Input: part model. Units: mm. Frame: model coordinates. Face numbers are marked on the shaded views. A direction names the side the tool comes from. Give positions to 0.01 mm unless a question says otherwise; leave off trailing zeros. Loops run counter-clockwise (first coordinate to the right, second up) from the corner with the lowest first, then second, coordinate; pieces in that order, holes last. Notation, with made-up numbers: (86.5, 51) - (139.5, 51) arc R23 cw to (139.5, 66) - close; hole circle Ø1 at (-29.75, 35). An arc over 180 degrees is marked (long way). One line per item, written item: value.
from build123d import *

# Parameters (mm, degrees)
SKETCH_1_W             = 80
SKETCH_1_H             = 80
EXTRUDE_1_DEPTH        = 12
HOLE_WIZARD_M161_D     = 14
HOLE_WIZARD_M161_DEPTH = 12
SKETCH_12_R            = 4.5
CUT_EXTRUDE_1_DEPTH    = 13
SKETCH_13_R            = 7.5
CUT_EXTRUDE_2_DEPTH    = 9


with BuildPart() as part:
    # Эскиз1 → Бобышка-Вытянуть1 (new body)
    with BuildSketch(Plane(origin=(0, 0, 0), x_dir=(1, 0, 0), z_dir=(0, 1, 0))):
        Rectangle(SKETCH_1_W, SKETCH_1_H)
    extrude(amount=EXTRUDE_1_DEPTH)

    # Отверстие обработанное метчиком M161
    with Locations(Plane(origin=(0, 12, 0), x_dir=(1, 0, 0), z_dir=(0, 1, 0))):
        with Locations((0, 0)):
            Hole(HOLE_WIZARD_M161_D / 2, depth=HOLE_WIZARD_M161_DEPTH)

    # Эскиз12 → Вырез-Вытянуть1 (cut, through all)
    with BuildSketch(Plane(origin=(0, 12, 0), x_dir=(1, 0, 0), z_dir=(0, 1, 0))):
        with Locations(Location((-20, 20, 0), (0, 0, 270))):  # turned: the seam where the file's is
            Circle(SKETCH_12_R)
        with Locations(Location((20, 20, 0), (0, 0, 270))):  # turned: the seam where the file's is
            Circle(SKETCH_12_R)
        with Locations(Location((20, -20, 0), (0, 0, 270))):  # turned: the seam where the file's is
            Circle(SKETCH_12_R)
        with Locations(Location((-20, -20, 0), (0, 0, 270))):  # turned: the seam where the file's is
            Circle(SKETCH_12_R)
    extrude(amount=-CUT_EXTRUDE_1_DEPTH, mode=Mode.SUBTRACT)

    # Эскиз13 → Вырез-Вытянуть2 (cut)
    with BuildSketch(Plane(origin=(0, 12, 0), x_dir=(1, 0, 0), z_dir=(0, 1, 0))):
        with Locations(Location((-20, 20, 0), (0, 0, 270))):  # turned: the seam where the file's is
            Circle(SKETCH_13_R)
        with Locations(Location((20, 20, 0), (0, 0, 270))):  # turned: the seam where the file's is
            Circle(SKETCH_13_R)
        with Locations(Location((20, -20, 0), (0, 0, 270))):  # turned: the seam where the file's is
            Circle(SKETCH_13_R)
        with Locations(Location((-20, -20, 0), (0, 0, 270))):  # turned: the seam where the file's is
            Circle(SKETCH_13_R)
    extrude(amount=-CUT_EXTRUDE_2_DEPTH, mode=Mode.SUBTRACT)


solid = part.part
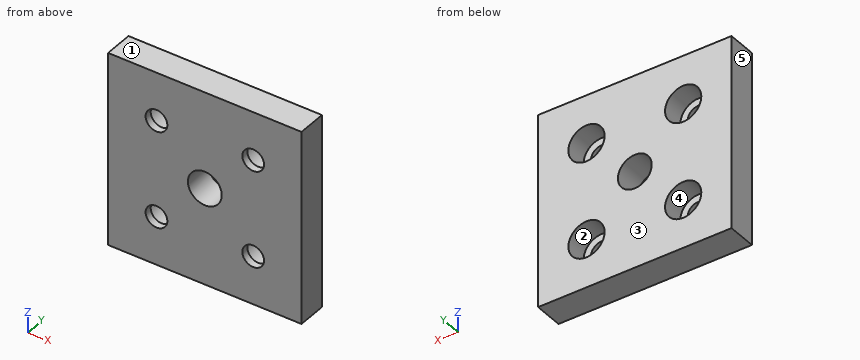
Item 1: Section A-A, the plane z = -20. Output: boundary loops of the cut face in (x, y).
Verdict:
outline: (-40, 0) - (-24.5, 0) - (-24.5, 3) - (-27.5, 3) - (-27.5, 12) - (-40, 12) - close; (-15.5, 0) - (15.5, 0) - (15.5, 3) - (12.5, 3) - (12.5, 12) - (-12.5, 12) - (-12.5, 3) - (-15.5, 3) - close; (24.5, 0) - (40, 0) - (40, 12) - (27.5, 12) - (27.5, 3) - (24.5, 3) - close
Item 2: Pin query (flat end, axial travel): P1, Ø4.5, axis at x = -23, z = 16.5, coming from the +Y side; P2, Ø1, axis at x = -3.5, z = 27.5, coming from the -Y side. Return the tip coordinate at first contact, or that it passes through.
Verdict:
P1: stops at y = 3
P2: stops at y = 0
Item 3: Section D-D, the plane z = 0. Output: boundary loops of the cut face in (x, y), and give its area (3 significant figures).
Verdict:
outline: (-40, 0) - (-7, 0) - (-7, 12) - (-40, 12) - close; (7, 0) - (40, 0) - (40, 12) - (7, 12) - close
area: 792 mm^2
Item 4: Section B-B, the plane x = 20. Output: boundary loops of the cut face in (y, z).
Verdict:
outline: (0, -40) - (12, -40) - (12, -27.5) - (3, -27.5) - (3, -24.5) - (0, -24.5) - close; (0, -15.5) - (3, -15.5) - (3, -12.5) - (12, -12.5) - (12, 12.5) - (3, 12.5) - (3, 15.5) - (0, 15.5) - close; (0, 24.5) - (3, 24.5) - (3, 27.5) - (12, 27.5) - (12, 40) - (0, 40) - close
Item 5: Section C-C, the plane y = 6. Output: boundary loops of the cut face in (x, z), and give its area (3 significant figures).
Verdict:
outline: (-40, -40) - (40, -40) - (40, 40) - (-40, 40) - close; hole circle Ø15 at (-20, -20); hole circle Ø15 at (-20, 20); hole circle Ø14 at (0, 0); hole circle Ø15 at (20, -20); hole circle Ø15 at (20, 20)
area: 5,540 mm^2
Item 6: Material intervals for L1, parallel to X at y = 5.25, z = -20; L2, parallel to Z at x = 26, y = 7.5, sorted ascending.
Verdict:
L1: x = -40 to -27.5, -12.5 to 12.5, 27.5 to 40
L2: z = -40 to -24.5, -15.5 to 15.5, 24.5 to 40
Item 7: Access query for the marked faces 4 and 5. Directions: +Z, -Z, +X, -X, +Y, -Y. A direction counts if a zero-diameter tool reaches every point of the face in a straight line with its end or side. Return the directions, or none.
Verdict:
face 4: +Y
face 5: +Z, -Z, -X, +Y, -Y
Item 8: Draft query along Z for the marked faces 1, 2 and 3. Return one class per face: pulls with the +Z half, pulls with the -Z half, needs draft (parallel to the pull), parting line crosses it, or undercut.
Verdict:
face 1: pulls with the +Z half
face 2: undercut
face 3: needs draft
